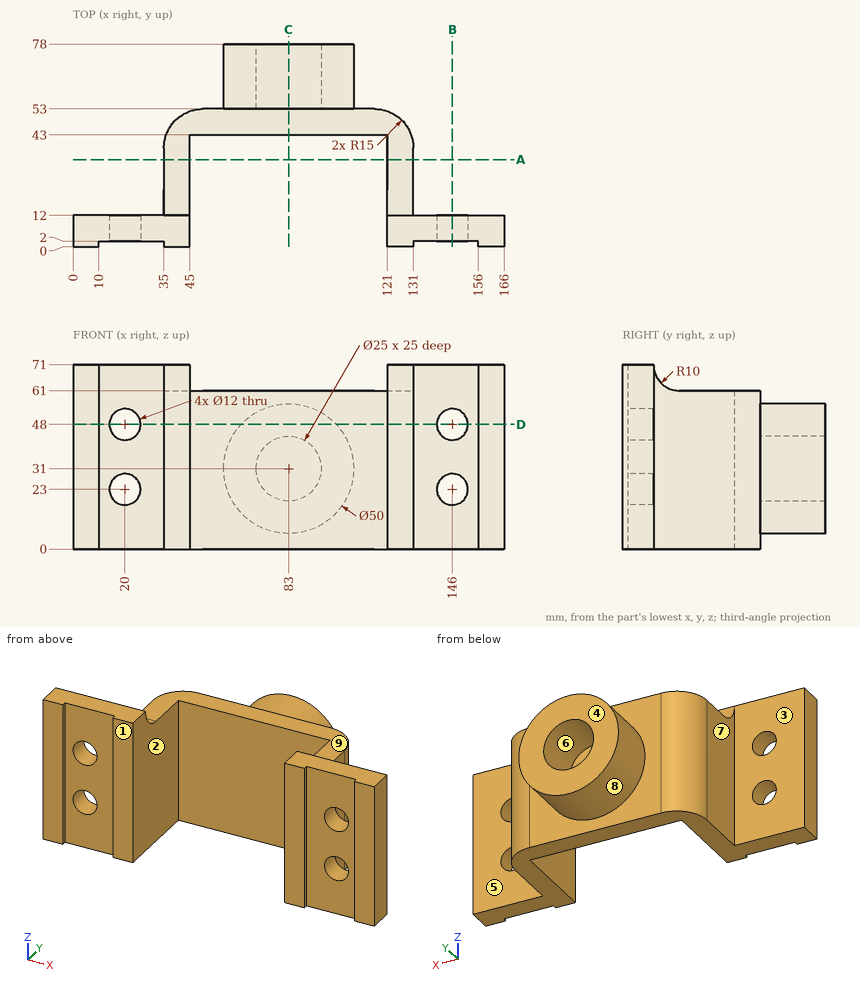
Study the drawing (mm; zero at the part's minimum x, y, z) and answer. A direction names the side the tool comes from. Coordinates: 2 decimals unless noted, no trailing zeros. Write each loop counter-clockwise with the first axis right and the second up, starting at its lowest first coordinate (ties: lowest second). Pieces come first, ordered by that corner, then holes. Notation, with made-up numbers: (48.25, 37) -> (84.25, 37) arc R18 cw to (84.25, 49) -> close; hole circle Ø2 at (-14, -18.75). An arc over 180 degrees is marked (long way). Write each question's results on one line, items separated by ' | '. Start each with the question number.
1) For a pull along Z with two mould halves and no side action, classify the marked faces 6, 7, 8 and 9 as +Z half, -Z half, draft (parallel to the pull), parting line (faces both ways), or undercut.
2) A cutting plane is placed at D-D (z = 48). Count the separate pieces of the cut face and the enclosed holes in it, then the cut area to 3 significant figures.
3) A cutting plane is placed at A-A (y = 33.5). Determine the outline of the cut face in (x, z).
4) A tool of negligible diameter and unlimited length cuts with its end or side. For the marked faces 1, 2, 3, 4 and 5, from which of +Z, -Z, +X, -X, +Y, -Y can it reach the whole face along a straight path? Write none if from no direction.
5) Flat-ended cylindrical pins translate along their axes: pin 1 Ø1.5 at (y, z) = (35.5, 23) entering from -X; pin 2 Ø21 at (y, z) = (29.5, 49.5) entering from +X; pin 3 Ø12 at (y, z) = (12.5, 22.5) entering from -X; pin 4 Ø18.5 at (x, z) = (100.5, 33.5) entering from -Y. Find the tip coordinate at first contact, or state that the pin passes through.
6) A cutting plane is placed at C-C (x = 83). Determine the outline of the cut face in (y, z), then the cut area to 4 significant figures.
7) A cutting plane is placed at B-B (x = 146). Determine the outline of the cut face in (y, z), then the cut area to 3 significant figures.
8) Straight lines are drawn through the part: probe 1 along X at (y, z) = (7, 23); probe 2 along Z at (x, y) = (146, 5.25); probe 3 along X at (y, z) = (24.5, 52). For each, find the intervals that lie inside material, in ascending order.
Values follow:
1) face 6: undercut | face 7: draft | face 8: parting line | face 9: +Z half
2) separate pieces: 3 | enclosed holes: 0 | area: 3,140 mm²
3) outline: (35, 0) -> (45, 0) -> (45, 61) -> (35, 61) -> close; (121, 0) -> (131, 0) -> (131, 61) -> (121, 61) -> close
4) face 1: +Z, -Z, +X, -X, -Y | face 2: +Z, -Z, -Y | face 3: +Z, -Z, -X, +Y | face 4: +Z, -Z, +X, -X, +Y | face 5: +Z, -Z, +X, +Y
5) pin 1: x = 35 | pin 2: x = 131 | pin 3: x = 0 | pin 4: y = 43
6) outline: (43, 0) -> (53, 0) -> (53, 6) -> (78, 6) -> (78, 18.5) -> (53, 18.5) -> (53, 43.5) -> (78, 43.5) -> (78, 56) -> (53, 56) -> (53, 61) -> (43, 61) -> close | area: 1,235 mm²
7) outline: (2, 0) -> (12, 0) -> (12, 17) -> (2, 17) -> close; (2, 29) -> (12, 29) -> (12, 42) -> (2, 42) -> close; (2, 54) -> (12, 54) -> (12, 71) -> (2, 71) -> close | area: 470 mm²
8) probe 1: 0 to 14, 26 to 45, 121 to 140, 152 to 166 | probe 2: 0 to 17, 29 to 42, 54 to 71 | probe 3: 35 to 45, 121 to 131
